```python
from build123d import *

# Parameters (mm, degrees)
F0_R      = 19.05
F1_DEPTH  = 109.474
F2_R      = 15.873592274
F3_DEPTH  = 109.728
F4_R      = 19.05
F5_DEPTH  = 1.27
F25_DEPTH = 25.4
F26_DEPTH = 32.004
F28_DEPTH = 45.466
F30_DEPTH = 34.036
F32_DEPTH = 25.4
F34_DEPTH = 25.4
F36_DEPTH = 53.086
F38_DEPTH = 65.786
F39_R     = 19.05
F40_DEPTH = 4.826
F41_R     = 16.1364398947
F41_R_2   = 15.139722271
F42_DEPTH = 1.27
F43_SIZE  = 0.254
F44_R     = 8.561127958
F44_R_2   = 8.1224197416
F45_DEPTH = 0.508


with BuildPart() as f1:
    # F0 (on Top) → F1 (new body)
    with BuildSketch(Plane.XY):
        Circle(F0_R)
    extrude(amount=F1_DEPTH)

    # F2 (on face) → F3 (cut)
    with BuildSketch(Plane.XY.offset(109.474)):
        Circle(F2_R)
    extrude(amount=-F3_DEPTH, mode=Mode.SUBTRACT)

    # F4 (on Top) → F5 (join)
    with BuildSketch(Plane.XY):
        Circle(F4_R)
    extrude(amount=-F5_DEPTH)

    # F24 (on face) → F25 (join)
    with BuildSketch(Plane(origin=(0, 0, 0), x_dir=(0.4275550934, 0.9039892931, 0), z_dir=(0.9039892931, -0.4275550934, 0))):
        with BuildLine():
            ThreePointArc((0, 70.5485), (2.595294019, 71.623505981), (3.6703, 74.2188))
            ThreePointArc((3.6703, 74.2188), (-2.595294019, 76.814094019), (0, 70.5485))
        make_face()
    extrude(amount=F25_DEPTH)

    # F26 (cut): a face of the model
    f26_faces = [f1.faces().sort_by_distance(p)[0] for p in [
        (22.9613280453, -10.8598993731, 74.2188),
    ]]
    extrude(f26_faces, amount=-F26_DEPTH, mode=Mode.SUBTRACT)

    # F27 (on face) → F28 (cut)
    with BuildSketch(Plane(origin=(0, 0, 0), x_dir=(-0.4275550934, 0.9039892931, 0), z_dir=(0.9039892931, 0.4275550934, 0))):
        with BuildLine():
            ThreePointArc((0, 70.5485), (2.595294019, 71.623505981), (3.6703, 74.2188))
            ThreePointArc((3.6703, 74.2188), (-2.595294019, 76.814094019), (0, 70.5485))
        make_face()
    extrude(amount=F28_DEPTH, mode=Mode.SUBTRACT)

    # F29 (on face) → F30 (cut)
    with BuildSketch(Plane(origin=(0, 0, 0), x_dir=(0.9700312532, -0.2429801799, 0), z_dir=(-0.2429801799, -0.9700312532, 0))):
        with BuildLine():
            ThreePointArc((0, 70.5485), (2.595294019, 71.623505981), (3.6703, 74.2188))
            ThreePointArc((3.6703, 74.2188), (-2.595294019, 76.814094019), (0, 70.5485))
        make_face()
    extrude(amount=-F30_DEPTH, mode=Mode.SUBTRACT)

    # F31 (on face) → F32 (cut)
    with BuildSketch(Plane(origin=(0, 0, 0), x_dir=(0.7730104534, 0.6343932842, 0), z_dir=(0.6343932842, -0.7730104534, 0))):
        with BuildLine():
            ThreePointArc((0, 70.5485), (2.595294019, 71.623505981), (3.6703, 74.2188))
            ThreePointArc((3.6703, 74.2188), (-2.595294019, 76.814094019), (0, 70.5485))
        make_face()
    extrude(amount=-F32_DEPTH, mode=Mode.SUBTRACT)

    # F33 (on Right) → F34 (cut)
    with BuildSketch(Plane.YZ):
        with BuildLine():
            ThreePointArc((0, 70.5485), (2.595294019, 71.623505981), (3.6703, 74.2188))
            ThreePointArc((3.6703, 74.2188), (-2.595294019, 76.814094019), (0, 70.5485))
        make_face()
    extrude(amount=-F34_DEPTH, mode=Mode.SUBTRACT)

    # F35 (on face) → F36 (cut)
    with BuildSketch(Plane(origin=(0, 0, 0), x_dir=(0.7730104534, -0.6343932842, 0), z_dir=(-0.6343932842, -0.7730104534, 0))):
        with BuildLine():
            ThreePointArc((0, 70.5485), (2.595294019, 71.623505981), (3.6703, 74.2188))
            ThreePointArc((3.6703, 74.2188), (-2.595294019, 76.814094019), (0, 70.5485))
        make_face()
    extrude(amount=F36_DEPTH, mode=Mode.SUBTRACT)

    # F37 (on face) → F38 (cut)
    with BuildSketch(Plane(origin=(0, 0, 0), x_dir=(0.9807852804, 0.195090322, 0), z_dir=(0.195090322, -0.9807852804, 0))):
        with BuildLine():
            ThreePointArc((0, 70.5485), (2.595294019, 71.623505981), (3.6703, 74.2188))
            ThreePointArc((3.6703, 74.2188), (-2.595294019, 76.814094019), (0, 70.5485))
        make_face()
    extrude(amount=F38_DEPTH, mode=Mode.SUBTRACT)

    # F39 (on Top) → F40 (join)
    with BuildSketch(Plane.XY):
        Circle(F39_R)
    extrude(amount=-F40_DEPTH)

    # F41 (on face) → F42 (cut)
    with BuildSketch(Plane(origin=(0, 0, -4.826), x_dir=(1, 0, 0), z_dir=(0, 0, -1))):
        Circle(F41_R)
        Circle(F41_R_2, mode=Mode.SUBTRACT)
    extrude(amount=-F42_DEPTH, mode=Mode.SUBTRACT)

    # F43
    f43_edges = [f1.edges().sort_by_distance(p)[0] for p in [
        (-15.139722, 0, -3.556),
    ]]
    chamfer(f43_edges, length=F43_SIZE)

    # F44 (on face) → F45 (cut)
    with BuildSketch(Plane(origin=(0, 0, -4.826), x_dir=(1, 0, 0), z_dir=(0, 0, -1))):
        Circle(F44_R)
        Circle(F44_R_2, mode=Mode.SUBTRACT)
    extrude(amount=-F45_DEPTH, mode=Mode.SUBTRACT)


solid = f1.part
```
Geometry check sheet. Reference: the model listing, model coordinates, mm. A direction names the side the tool comes from. Coordinates: 2 decimals unless noted, no trailing zeros. Loops run counter-clockwise (first coordinate to the right, second up) from the corner with the lowest first, then second, coordinate; pieces in that order, holes last.
Item 1: Thickness scan on line 1 (Y direction, x = 0, z = -3.8); line 2 (X direction, y = 0, z = 80.5). Record the ranges inside material, lowest first.
Item 2: Sectioned sample at A-A, the plane z = 89. Record the boundary of the cut face in (x, y).
Item 3: Release check for a two-part mould opening along Y. For faces 4 (the face through (0, 0, 0)), 5 (the face through (7, -7, -4.826)), 6 (the face through (-15.12, -11.59, 53.12)) record: released by +Y, released by -Y, zero draft, split by the parting line, or undercut.
Item 4: Go/stop test with flat-tipped pins: pin 1 Ø1.5 at (y, z) = (13.5, 46) entering from -X; pin 2 Ø1 at (y, z) = (-14, 57.5) entering from +X; pin 3 Ø9.5 at (x, y) = (3.5, -6) entering from +Z. Record where each tip stops, or that it passes through.
Item 5: Access from +Z, -Z, +X, -X, +Y, -Y to the whole of each face (thin tool, end or side, straight path). Record for faces 1 (the face through (-16, 4, -4.826)), 2 (the face through (6.99, 13.43, -4.33)), 3 (the face through (-12.597, -9.659, 55.503)).
Check result:
1. line 1: y = -19.05 to -16.14, -15.15 to 15.15, 16.14 to 19.05
1. line 2: x = -19.05 to -15.87, 15.87 to 19.05
2. outline: circle Ø38.1 at (0, 0); hole circle Ø31.75 at (0, 0)
3. face 4: undercut
3. face 5: zero draft
3. face 6: split by the parting line
4. pin 1: stops at x = -14.15
4. pin 2: stops at x = 13.44
4. pin 3: stops at z = 0
5. face 1: -Z, +X, -X, +Y, -Y
5. face 2: -Z
5. face 3: +Z
